The model under review builds one solid part; all positions refer to its coordinate system, in mm. Face numbers are marked on the shaded views. Give positions to 0.01 mm unless a question says otherwise; leave off trailing zeros. Order: outer loops, then holes, each group sorted by start corner. A loop starts at its lowest first (then second) coordinate and runs counter-clockwise, first axis right, second up. Notation, with made-up numbers: (83, 86.25) - (96, 86.25) arc R22 cw to (96, 113.25) - close; hole circle Ø10 at (68, 49.25). An arc over 180 degrees is marked (long way). Use CSV: the item, a comma, the result in double quotes. Start each with the question number.
1. Take a section at C-C, the plane y = 17.5. State the section outline as (x, z) points (3 decimals), then the cut area to 3 significant figures.
2. Take a section at A-A, the plane z = -1.25. State the section outline as (x, y) points (3 decimals), then the cut area to 3 significant figures.
3. Draft analysis for pull direction Y (two halves, no side actions). For the marked faces 1, 2 and 3, state which applies: released by +Y, released by -Y, zero draft, split by the parting line, or undercut.
4. Take a section at B-B, the plane x = 27.5. State the section outline as (y, z) points.
5. To check wall thickness, follow line 1 (Y direction, x = 20, z = 1.25); line 2 (X direction, y = -1, z = 2.25) (3 decimals); line 3 (X direction, y = 15, z = 0) (3 decimals). State the ranges of each line that lie inside material, in increasing order. Write a range as [from, to].
6. For pin 1 (1 mm diameter, centred on x = 13.5, z = 1.5, fed in from +Y); pin 2 (3 mm diameter, centred on y = 10.5, z = -4.5, fed in from -X); pin 3 (4 mm diameter, centred on x = 21, z = 2.5, fed in from -Y), all flat-tipped, find the tip position at first contact; note any pin that passes through.
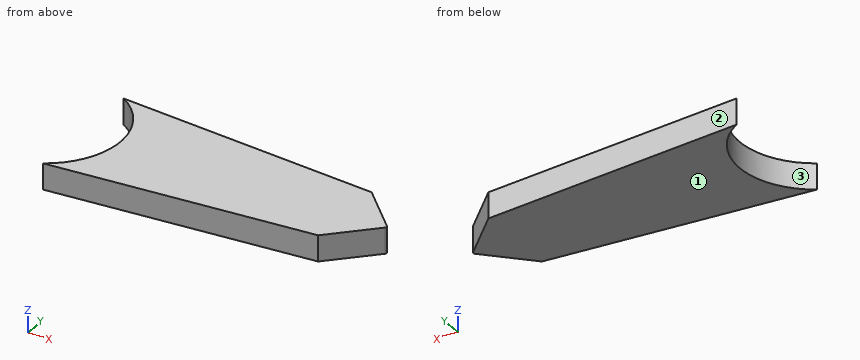
```python
from build123d import *

# Parameters (mm, degrees)
BOSS_EXTRUDE1_DEPTH = 6
FILLET1_R           = 1


with BuildPart() as part:
    # Sketch1 → Boss-Extrude1 (new, symmetric)
    with BuildSketch(Plane.XY):
        with BuildLine():
            Line((51.083153784, -19.901846216), (-70.987243623, -30))
            ThreePointArc((-70.987243623, -30), (-54.015, 0), (-70.987243623, 30))
            Line((-70.987243623, 30), (51.083153784, 19.901846216))
            Line((51.083153784, 19.901846216), (70.985, 0))
            Line((70.985, 0), (51.083153784, -19.901846216))
        make_face()
    extrude(amount=BOSS_EXTRUDE1_DEPTH, both=True)

    # Fillet1
    fillet1_edges = [part.edges().sort_by_distance(p)[0] for p in [
        (70.985, 0, 0),
    ]]
    fillet(fillet1_edges, radius=FILLET1_R)


solid = part.part
```
Determined:
1,outline,"(-58.704, -6) - (53.485, -6) - (53.485, 6) - (-58.704, 6) - close"
1,area,"1,350 mm²"
2,outline,"(-70.987, -30) - (51.083, -19.902) - (70.278, -0.707) arc R1 ccw to (70.278, 0.707) - (51.083, 19.902) - (-70.987, 30) arc R35 cw to start"
2,area,"5,770 mm²"
3,face 1,"zero draft"
3,face 2,"released by +Y"
3,face 3,"undercut"
4,outline,"(-21.85, -6) - (21.85, -6) - (21.85, 6) - (-21.85, 6) - close"
5,line 1,"y = [-22.47, 22.47]"
5,line 2,"x = [-54.029, 69.985]"
5,line 3,"x = [-57.392, 55.985]"
6,pin 1,"stops at y = 23.05"
6,pin 2,"stops at x = -56.14"
6,pin 3,"stops at y = -22.56"
